CAD build for the part. Positions are in the model's coordinates, mm. A direction names the side the tool comes from. Round coordinates to 2 decimals unless told otherwise and drop trailing zeros. Loops run counter-clockwise (first coordinate to the right, second up) from the corner with the lowest first, then second, coordinate; pieces in that order, holes last.
```python
from build123d import *

# Parameters (mm, degrees)
SKIZZE1_W                                    = 56
SKIZZE1_H                                    = 86
AUFSATZ_LINEAR_AUSTRAGEN1_DEPTH              = 22
WANDUNG1_T                                   = -2
SKIZZE2_R                                    = 4.5
AUFSATZ_LINEAR_AUSTRAGEN2_DEPTH              = 4
VERRUNDUNG1_R                                = 2
STIRNSENKUNG_F_R_M3_ZYLINDERSCHRAUBE_2_COUNT = 2
STIRNSENKUNG_F_R_M3_ZYLINDERSCHRAUBE_2_PITCH = 81.987803971
STIRNSENKUNG_F_R_M3_ZYLINDERSCHRAUBE_3_COUNT = 2
STIRNSENKUNG_F_R_M3_ZYLINDERSCHRAUBE_3_PITCH = 71
STIRNSENKUNG_F_R_M3_ZYLINDERSCHRAUBE_4_COUNT = 2
STIRNSENKUNG_F_R_M3_ZYLINDERSCHRAUBE_4_PITCH = 41
SKIZZE8_W                                    = 39.14
SKIZZE8_H                                    = 12.26
SCHNITT_LINEAR_AUSTRAGEN3_DEPTH              = 10
VERRUNDUNG2_R                                = 3
SKIZZE9_W                                    = 30.81
SKIZZE9_H                                    = 12.87
SCHNITT_LINEAR_AUSTRAGEN4_DEPTH              = 10
VERRUNDUNG3_R                                = 3
SKIZZE10_R                                   = 2
SCHNITT_LINEAR_AUSTRAGEN5_DEPTH              = 10
SKIZZE11_W                                   = 14
SKIZZE11_H                                   = 16
AUFSATZ_LINEAR_AUSTRAGEN3_DEPTH              = 4
VERRUNDUNG4_R                                = 3
SPIEGELN1_OUTLINE_R                          = 3.3
SPIEGELN1_DEPTH                              = 4


with BuildPart() as part:
    # Skizze1 → Aufsatz-Linear austragen1 (new body)
    with BuildSketch(Plane(origin=(0, 0, 0), x_dir=(1, 0, 0), z_dir=(0, 1, 0))):
        with Locations((28, 43)):
            Rectangle(SKIZZE1_W, SKIZZE1_H)
    extrude(amount=AUFSATZ_LINEAR_AUSTRAGEN1_DEPTH)

    # Wandung1
    wandung1_openings = [part.faces().sort_by_distance(p)[0] for p in [
        (28, 22, -43),
    ]]
    offset(amount=WANDUNG1_T, openings=wandung1_openings, kind=Kind.INTERSECTION)

    # Skizze2 → Aufsatz-Linear austragen2 (add)
    with BuildSketch(Plane(origin=(0, 2, 0), x_dir=(1, 0, 0), z_dir=(0, 1, 0))):
        with Locations(Location((7.5, 7.5, 0), (0, 0, 90))):
            Circle(SKIZZE2_R)
        with Locations(Location((48.5, 7.5, 0), (0, 0, 90))):
            Circle(SKIZZE2_R)
        with Locations(Location((48.5, 78.5, 0), (0, 0, 90))):
            Circle(SKIZZE2_R)
        with Locations(Location((7.5, 78.5, 0), (0, 0, 90))):
            Circle(SKIZZE2_R)
    extrude(amount=AUFSATZ_LINEAR_AUSTRAGEN2_DEPTH)

    # Verrundung1
    verrundung1_edges = [part.edges().sort_by_distance(p)[0] for p in [
        (0, 11, -86),
        (56, 11, -86),
        (56, 11, 0),
        (0, 11, 0),
    ]]
    fillet(verrundung1_edges, radius=VERRUNDUNG1_R)

    # Skizze6 → Stirnsenkung für M3 Zylinderschraube mit Innensechskant1 (revolve, cut)
    with BuildSketch(Plane(origin=(48.5, 0, -7.5), x_dir=(0, 0, -1), z_dir=(1, 0, 0))):
        Polygon((0, 0), (0, 15.021463052), (1.7, 14), (1.7, 3.4), (3.25, 3.4), (3.25, 0.025), (3.275, 0), align=None)
    stirnsenkung_f_r_m3_zylinderschraube_mit = revolve(axis=Axis((48.5, -6.35, -7.5), (0, 1, 0)), mode=Mode.SUBTRACT)

    # Stirnsenkung f_r M3 Zylinderschraube 2: Stirnsenkung für M3 Zylinderschraube mit Innensechskant1 ×2
    with Locations(*[Vector(-0.5000743770922673, 0, -0.865982457891487) * (i * STIRNSENKUNG_F_R_M3_ZYLINDERSCHRAUBE_2_PITCH) for i in range(1, STIRNSENKUNG_F_R_M3_ZYLINDERSCHRAUBE_2_COUNT)]):
        add(stirnsenkung_f_r_m3_zylinderschraube_mit, mode=Mode.SUBTRACT)

    # Stirnsenkung f_r M3 Zylinderschraube 3: Stirnsenkung für M3 Zylinderschraube mit Innensechskant1 ×2
    with Locations(*[(0, 0, -i * STIRNSENKUNG_F_R_M3_ZYLINDERSCHRAUBE_3_PITCH) for i in range(1, STIRNSENKUNG_F_R_M3_ZYLINDERSCHRAUBE_3_COUNT)]):
        add(stirnsenkung_f_r_m3_zylinderschraube_mit, mode=Mode.SUBTRACT)

    # Stirnsenkung f_r M3 Zylinderschraube 4: Stirnsenkung für M3 Zylinderschraube mit Innensechskant1 ×2
    with Locations(*[(-i * STIRNSENKUNG_F_R_M3_ZYLINDERSCHRAUBE_4_PITCH, 0, 0) for i in range(1, STIRNSENKUNG_F_R_M3_ZYLINDERSCHRAUBE_4_COUNT)]):
        add(stirnsenkung_f_r_m3_zylinderschraube_mit, mode=Mode.SUBTRACT)

    # Skizze8 → Schnitt-Linear austragen3 (cut)
    with BuildSketch(Plane(origin=(56, 0, 0), x_dir=(0, 0, -1), z_dir=(1, 0, 0))):
        with Locations((43, 15.87)):
            Rectangle(SKIZZE8_W, SKIZZE8_H)
    extrude(amount=-SCHNITT_LINEAR_AUSTRAGEN3_DEPTH, mode=Mode.SUBTRACT)

    # Verrundung2
    verrundung2_edges = [part.edges().sort_by_distance(p)[0] for p in [
        (55, 9.74, -23.43),
        (55, 9.74, -62.57),
    ]]
    fillet(verrundung2_edges, radius=VERRUNDUNG2_R)

    # Skizze9 → Schnitt-Linear austragen4 (cut)
    with BuildSketch(Plane(origin=(2, 0, 0), x_dir=(0, 0, -1), z_dir=(1, 0, 0))):
        with Locations((43.285, 15.565)):
            Rectangle(SKIZZE9_W, SKIZZE9_H)
    extrude(amount=-SCHNITT_LINEAR_AUSTRAGEN4_DEPTH, mode=Mode.SUBTRACT)

    # Verrundung3
    verrundung3_edges = [part.edges().sort_by_distance(p)[0] for p in [
        (1, 9.13, -27.88),
        (1, 9.13, -58.69),
    ]]
    fillet(verrundung3_edges, radius=VERRUNDUNG3_R)

    # Skizze10 → Schnitt-Linear austragen5 (cut)
    with BuildSketch(Plane(origin=(0, 0, -86), x_dir=(-1, 0, 0), z_dir=(0, 0, -1))):
        with Locations((-41.5, 12.7)):
            Circle(SKIZZE10_R)
        with Locations((-33.5, 12.7)):
            Circle(SKIZZE10_R)
        with Locations((-25.95, 11.62)):
            Circle(SKIZZE10_R)
        with Locations((-15.95, 11.62)):
            Circle(SKIZZE10_R)
    extrude(amount=-SCHNITT_LINEAR_AUSTRAGEN5_DEPTH, mode=Mode.SUBTRACT)

    # Skizze11 → Aufsatz-Linear austragen3 (add)
    with BuildSketch(Plane(origin=(0, 0, 0), x_dir=(1, 0, 0), z_dir=(0, 1, 0))):
        with Locations((28, 94)):
            Rectangle(SKIZZE11_W, SKIZZE11_H)
    extrude(amount=AUFSATZ_LINEAR_AUSTRAGEN3_DEPTH)

    # Verrundung4
    verrundung4_edges = [part.edges().sort_by_distance(p)[0] for p in [
        (35, 2, -86),
        (35, 2, -102),
        (21, 2, -102),
        (21, 2, -86),
    ]]
    fillet(verrundung4_edges, radius=VERRUNDUNG4_R)

    # Skizze13 → Durchgangsloch für M61 (revolve, cut)
    with BuildSketch(Plane(origin=(28, 4, -94), x_dir=(0, 0, 1), z_dir=(1, 0, 0))):
        Polygon((0, 0), (0, 15.982840043), (3.3, 14), (3.3, 0.025), (3.325, 0), align=None)
    revolve(axis=Axis((28, 10.35, -94), (0, -1, 0)), mode=Mode.SUBTRACT)

    # Spiegeln1: read off the stored shape, not the designer's step
    # Spiegeln1 outline → Spiegeln1 (add)
    with BuildSketch(Plane(origin=(0, 0, 0), x_dir=(1, 0, 0), z_dir=(0, 1, 0))):
        with BuildLine():
            ThreePointArc((32, -16), (34.121320344, -15.121320344), (35, -13))
            Line((35, -13), (35, 0))
            Line((35, 0), (21, 0))
            Line((21, 0), (21, -13))
            ThreePointArc((21, -13), (21.878679656, -15.121320344), (24, -16))
            Line((24, -16), (32, -16))
        make_face()
        with Locations((28, -8)):
            Circle(SPIEGELN1_OUTLINE_R, mode=Mode.SUBTRACT)
    extrude(amount=SPIEGELN1_DEPTH)

    # Spiegeln1 2 outline → Spiegeln1 2 (revolve, cut)
    with BuildSketch(Plane(origin=(28, 0, 8), x_dir=(1, 0, 0), z_dir=(0, 0, 1))):
        Polygon((3.3, 4), (3.3, 3.975), (3.325, 4), align=None)
    revolve(axis=Axis((28, 0, 8), (0, 1, 0)), mode=Mode.SUBTRACT)


solid = part.part
```
Item 1: Cut at A-A, the plane z = 8. Give the cut face in (x, y) (3 decimals).
Answers follow:
outline: (21, 0) - (24.7, 0) - (24.7, 3.975) - (24.675, 4) - (21, 4) - close; (31.3, 0) - (35, 0) - (35, 4) - (31.325, 4) - (31.3, 3.975) - close
Item 2: Probe line 1 (Z direction, x = 48.5, y = 4.8); line 2 (X direction, y = 4.95, z = -78.5); line 3 (X direction, y = 1.6, z = -7.5). List the from-to ranges inside material, lowest first.
Answers follow:
line 1: z = -86 to -84, -83 to -80.2, -76.8 to -74, -12 to -9.2, -5.8 to -3, -2 to 0
line 2: x = 0 to 2, 3 to 5.8, 9.2 to 12, 44 to 46.8, 50.2 to 53, 54 to 56
line 3: x = 0 to 4.25, 10.75 to 45.25, 51.75 to 56
Item 3: Cut at D-D, the plane y = 18.75. Give the cut face in (x, z).
Answers follow:
outline: (0, -84) arc R2 ccw to (2, -86) - (54, -86) arc R2 ccw to (56, -84) - (56, -62.57) - (54, -62.57) - (54, -84) - (2, -84) - (2, -58.69) - (0, -58.69) - close; (0, -27.88) - (2, -27.88) - (2, -2) - (54, -2) - (54, -23.43) - (56, -23.43) - (56, -2) arc R2 ccw to (54, 0) - (2, 0) arc R2 ccw to (0, -2) - close
Item 4: Flat gauge pins, fed straight in: P1, Ø2, axis at y = 1.5, z = -95.5, coming from the -X side; P2, Ø2, axis at x = 46, y = 10, coming from the -Z side; P3, Ø0.6, axis at x = 1, z = -47, coming from the +Y side. Where does each tip first touch, or does it go through?
Answers follow:
P1: stops at x = 21
P2: stops at z = -86
P3: stops at y = 9.13
Item 5: Cut at C-C, the plane x = 15.95. Give the cut face in (y, z).
Answers follow:
outline: (0, -86) - (9.62, -86) - (9.62, -84) - (2, -84) - (2, -2) - (22, -2) - (22, 0) - (0, 0) - close; (13.62, -86) - (22, -86) - (22, -84) - (13.62, -84) - close
Item 6: 3-axis set-ups, long thin cutter, end or side, ignore diameter. For faces 1 (the cylindrical face through (52.89, 3.97, -77.52)), 2 (the flat face through (50, 3.4, -6)), 3 (the flat face through (1, 9.13, -43)): which of +Z, -Z, +X, -X, +Y, -Y reach the whole face in a straight line?
Answers follow:
face 1: +Y
face 2: -Y
face 3: -X, +Y
Item 7: Cut at B-B, the plane y = 7.5. Give the cut face in (x, z).
Answers follow:
outline: (0, -84) arc R2 ccw to (2, -86) - (54, -86) arc R2 ccw to (56, -84) - (56, -2) arc R2 ccw to (54, 0) - (2, 0) arc R2 ccw to (0, -2) - close; hole (2, -84) - (54, -84) - (54, -2) - (2, -2) - close
